```python
from build123d import *

# Parameters (mm, degrees)
SKETCH1_R           = 2.5
SKETCH1_R_2         = 2.4892
SKETCH1_R_3         = 2.0701
BOSS_EXTRUDE1_DEPTH = 2.54


with BuildPart() as part:
    # Sketch1 → Boss-Extrude1 (new body)
    with BuildSketch(Plane.XY):
        with BuildLine():
            Line((85.66, -50.8), (65.34, -50.8))
            ThreePointArc((65.34, -50.8), (45.583436534, -58.983436534), (37.4, -78.74))
            Line((37.4, -78.74), (37.4, -93.98))
            ThreePointArc((37.4, -93.98), (36.656051224, -95.776051224), (34.86, -96.52))
            Line((34.86, -96.52), (14.54, -96.52))
            ThreePointArc((14.54, -96.52), (12.743948776, -95.776051224), (12, -93.98))
            Line((12, -93.98), (12, -50.8))
            Line((12, -50.8), (12, -27.94))
            ThreePointArc((12, -27.94), (12.743948776, -26.143948776), (14.54, -25.4))
            Line((14.54, -25.4), (85.66, -25.4))
            ThreePointArc((85.66, -25.4), (87.456051224, -26.143948776), (88.2, -27.94))
            Line((88.2, -27.94), (88.2, -48.26))
            ThreePointArc((88.2, -48.26), (87.456051224, -50.056051224), (85.66, -50.8))
        make_face()
        with Locations((24.7, -88.9)):
            Circle(SKETCH1_R, mode=Mode.SUBTRACT)
        with Locations((24.7, -76.2)):
            Circle(SKETCH1_R, mode=Mode.SUBTRACT)
        with Locations((24.7, -63.5)):
            Circle(SKETCH1_R, mode=Mode.SUBTRACT)
        with Locations((24.7, -50.8)):
            Circle(SKETCH1_R, mode=Mode.SUBTRACT)
        with Locations((24.7, -38.1)):
            Circle(SKETCH1_R_2, mode=Mode.SUBTRACT)
        with Locations((50.1, -38.1)):
            Circle(SKETCH1_R_3, mode=Mode.SUBTRACT)
        with Locations((75.5, -38.1)):
            Circle(SKETCH1_R_3, mode=Mode.SUBTRACT)
    extrude(amount=BOSS_EXTRUDE1_DEPTH)


solid = part.part
```
Work out the finished part from the listing and answer in its coordinate system (mm). A direction names the side the tool comes from. Give positions to 0.01 mm unless a question says otherwise; leave off trailing zeros. Loops run counter-clockwise (first coordinate to the right, second up) from the corner with the lowest first, then second, coordinate; pieces in that order, holes last. Notation, with made-up numbers: (-6, -35) -> (27, -35) arc R35 ccw to (27, -1) -> close; hole circle Ø7 at (-11, 86.25). An arc over 180 degrees is marked (long way). One line per question, with ' | ' between items. Start each with the question number.
1) For faces 1 (the face through (87.436, -26.124, 1.252)), 2 (the face through (37.4, -86, 1)), determine the directions among +Z, -Z, +X, -X, +Y, -Y from which every point of the face is accessible in a straight line to the end or side of a thin tool.
2) Section A-A, the plane x = 75.5 is taken. Determine the outline of the cut face in (y, z).
3) Section C-C, the plane z = 1.25 is taken. Determine the outline of the cut face in (x, y), then the cut area to 3 significant figures.
4) Section D-D, the plane x = 24.7 is taken. Determine the outline of the cut face in (y, z), then the cut area to 3 significant figures.
5) Determine the mould class of faces 3 (the face through (87.476, -50.036, 1.252)), 4 (the face through (25, -96.52, 1)), 5 (the face through (24.37, -86.42, 1.25)) for opening direction X: +X half, -X half, draft (parallel to the pull), parting line (faces both ways), or undercut.
6) Section B-B, the plane y = -88.9 is taken. Determine the outline of the cut face in (x, z).
7) Each of these flat-tipped pins is pushed along its axis until it touches: pin 1 (8 mm diameter, centred on x = 24.7, y = -76.2, fed in from +Z); pin 2 (1.3 mm diameter, centred on x = 76, z = 1.5, fed in from -Y). Where does it stop, or does it pass through?
8) Straight lines are drawn through the part: L1, parallel to Y at x = 24.7, z = 1.35; L2, parallel to X at y = -40, z = 1.8; L3, parallel to X at y = -36.5, z = 0.2. For each, find the intervals that lie inside material, in ascending order.
Resolved:
1) face 1: +Z, -Z, +X, +Y | face 2: +Z, -Z, +X, -Y
2) outline: (-50.8, 0) -> (-40.17, 0) -> (-40.17, 2.54) -> (-50.8, 2.54) -> close; (-36.03, 0) -> (-25.4, 0) -> (-25.4, 2.54) -> (-36.03, 2.54) -> close
3) outline: (12, -93.98) arc R2.54 ccw to (14.54, -96.52) -> (34.86, -96.52) arc R2.54 ccw to (37.4, -93.98) -> (37.4, -78.74) arc R27.94 cw to (65.34, -50.8) -> (85.66, -50.8) arc R2.54 ccw to (88.2, -48.26) -> (88.2, -27.94) arc R2.54 ccw to (85.66, -25.4) -> (14.54, -25.4) arc R2.54 ccw to (12, -27.94) -> close; hole circle Ø5 at (24.7, -88.9); hole circle Ø5 at (24.7, -76.2); hole circle Ø5 at (24.7, -63.5); hole circle Ø5 at (24.7, -50.8); hole circle Ø4.98 at (24.7, -38.1); hole circle Ø4.14 at (50.1, -38.1); hole circle Ø4.14 at (75.5, -38.1) | area: 3,130 mm2
4) outline: (-96.52, 0) -> (-91.4, 0) -> (-91.4, 2.54) -> (-96.52, 2.54) -> close; (-86.4, 0) -> (-78.7, 0) -> (-78.7, 2.54) -> (-86.4, 2.54) -> close; (-73.7, 0) -> (-66, 0) -> (-66, 2.54) -> (-73.7, 2.54) -> close; (-61, 0) -> (-53.3, 0) -> (-53.3, 2.54) -> (-61, 2.54) -> close; (-48.3, 0) -> (-40.59, 0) -> (-40.59, 2.54) -> (-48.3, 2.54) -> close; (-35.61, 0) -> (-25.4, 0) -> (-25.4, 2.54) -> (-35.61, 2.54) -> close | area: 117 mm2
5) face 3: +X half | face 4: draft | face 5: undercut
6) outline: (12, 0) -> (22.2, 0) -> (22.2, 2.54) -> (12, 2.54) -> close; (27.2, 0) -> (37.4, 0) -> (37.4, 2.54) -> (27.2, 2.54) -> close
7) pin 1: z = 2.54 | pin 2: y = -50.8
8) L1: -96.52 to -91.4, -86.4 to -78.7, -73.7 to -66, -61 to -53.3, -48.3 to -40.59, -35.61 to -25.4 | L2: 12 to 23.09, 26.31 to 49.28, 50.92 to 74.68, 76.32 to 88.2 | L3: 12 to 22.79, 26.61 to 48.79, 51.41 to 74.19, 76.81 to 88.2
